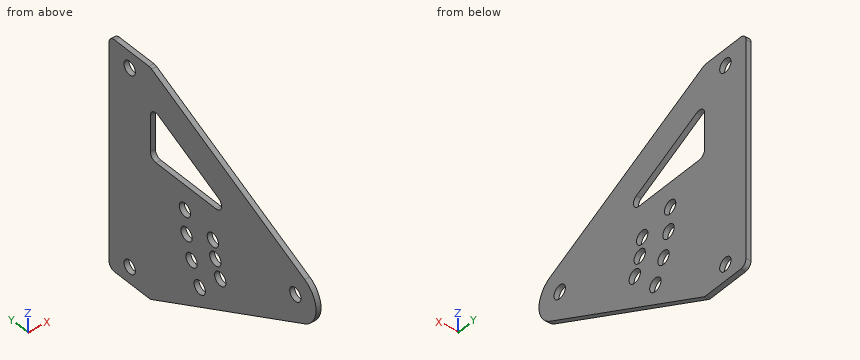
```python
from build123d import *

# Parameters (mm, degrees)
SKETCH_1_R      = 2.05
EXTRUDE_1_DEPTH = 1.5
FILLET_2_R      = 2


with BuildPart() as part:
    # ｽｹｯﾁ1 → ﾎﾞｽ - 押し出し1 (new body)
    with BuildSketch(Plane(origin=(0, 0, 0), x_dir=(0, 0, -1), z_dir=(1, 0, 0))):
        with BuildLine():
            Line((35, 67.5), (-35, 67.5))
            Line((-35, 67.5), (-35, 52.5))
            Line((-35, 52.5), (-6.690641581, -3.388999149))
            ThreePointArc((-6.690641581, -3.388999149), (0, -7.5), (6.690641581, -3.388999149))
            Line((6.690641581, -3.388999149), (35, 52.5))
            Line((35, 52.5), (35, 67.5))
        make_face()
        Circle(SKETCH_1_R, mode=Mode.SUBTRACT)
        with Locations((2.614672282, 29.885840943)):
            Circle(SKETCH_1_R, mode=Mode.SUBTRACT)
        with Locations((7.764571353, 28.977774789)):
            Circle(SKETCH_1_R, mode=Mode.SUBTRACT)
        with Locations((12.678547852, 27.189233611)):
            Circle(SKETCH_1_R, mode=Mode.SUBTRACT)
        Polygon((-7.5, 20.339282727), (-23.790312694, 52.5), (-7.5, 52.5), align=None, mode=Mode.SUBTRACT)
        with Locations((-30, 60)):
            Circle(SKETCH_1_R, mode=Mode.SUBTRACT)
        with Locations((13.680805733, 37.587704831)):
            Circle(SKETCH_1_R, mode=Mode.SUBTRACT)
        with Locations((0, 40)):
            Circle(SKETCH_1_R, mode=Mode.SUBTRACT)
        with Locations((6.945927107, 39.39231012)):
            Circle(SKETCH_1_R, mode=Mode.SUBTRACT)
        with Locations((20, 34.641016151)):
            Circle(SKETCH_1_R, mode=Mode.SUBTRACT)
        with Locations((30, 60)):
            Circle(SKETCH_1_R, mode=Mode.SUBTRACT)
    extrude(amount=EXTRUDE_1_DEPTH)

    # ﾌｨﾚｯﾄ2
    fillet_2_edges = [part.edges().sort_by_distance(p)[0] for p in [
        (0.75, 52.5, 35),
        (0.75, 67.5, 35),
        (0.75, 67.5, -35),
        (0.75, 52.5, -35),
        (0.75, 52.5, 23.790312694),
        (0.75, 20.339282727, 7.5),
        (0.75, 52.5, 7.5),
    ]]
    fillet(fillet_2_edges, radius=FILLET_2_R)


solid = part.part
```
Design review of the part built by this model. Coordinates are the model's own, in mm. Coordinates: 2 decimals unless noted, no trailing zeros. Order: outer loops, then holes, each group sorted by start corner. A loop starts at its lowest first (then second) coordinate and runs counter-clockwise, first axis right, second up. Notation, with made-up numbers: (38.5, -26) - (48.5, -26) arc R29 cw to (48.5, 9) - close; hole circle Ø5 at (-6.75, 67.25). An arc over 180 degrees is marked (long way). One line per question, with ' | ' between items.
Q1. Consider section B-B, the plane z = 17. Give the boundary of the cut face in (x, y).
Answer key:
outline: (0, 16.96) - (1.5, 16.96) - (1.5, 39.09) - (0, 39.09) - close; (0, 52.5) - (1.5, 52.5) - (1.5, 67.5) - (0, 67.5) - close
Q2. To check wall thickness, follow line 1 along Y through (x, z) = (1, -14.5); line 2 along Z through (x, y) = (0.7, 30); line 3 along Z through (x, y) = (0.25, 36). State the ranges of each line that lie inside material, in increasing order.
Answer key:
line 1: y = 12.03 to 26.25, 28.13 to 35.71, 39.47 to 67.5 | line 2: z = -23.6 to -9.54, -5.99 to -4.66, -0.57 to 7.5, 12.39 to 23.6 | line 3: z = -26.64 to -21.53, -18.47 to -14.98, -12.38 to 7.5, 15.43 to 26.64
Q3. Consider section C-C, the plane y = 13. Give the boundary of the cut face in (x, z).
Answer key:
outline: (0, -14.99) - (1.5, -14.99) - (1.5, 14.99) - (0, 14.99) - close
Q4. Clearance check with a flat-ended pin moving along its axis: pin 1 Ø2.5 at (y, z) = (34.64, -20) entering from -X. State where the tip first meets the part, or that it passes through.
Answer key:
pin 1: passes through
Q5. Consider section A-A, the plane y = 0. Give the boundary of the cut face in (x, z).
Answer key:
outline: (0, -8.41) - (1.5, -8.41) - (1.5, -2.05) - (0, -2.05) - close; (0, 2.05) - (1.5, 2.05) - (1.5, 8.41) - (0, 8.41) - close
